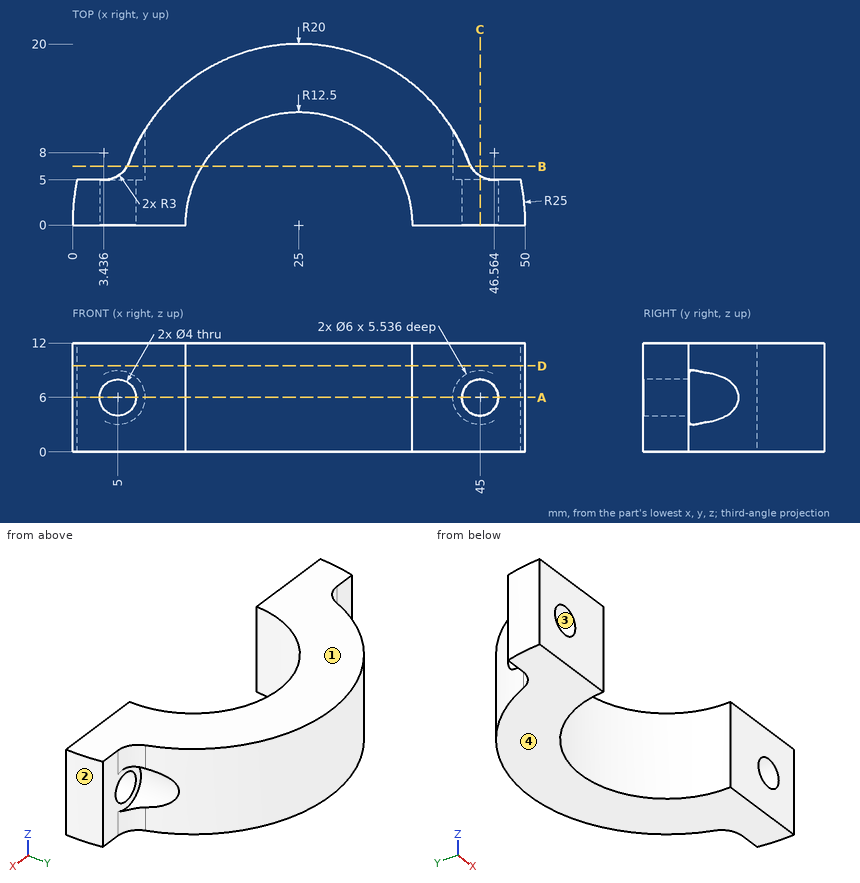
Could you check a few things on this drawing? It's one solid part, dimensions in mm from its lowest x, y, z. Coordinates: 2 decimals unless noted, no trailing zeros. Order: outer loops, then holes, each group sorted by start corner. A loop starts at its lowest first (then second) coordinate and runs counter-clockwise, first axis right, second up. Notation, with made-up numbers: (7, 40.25) -> (41, 40.25) arc R29 cw to (41, 70.25) -> close; hole circle Ø11 at (7, -39). An arc over 180 degrees is marked (long way). One line per item, written item: value. Start each with the question number.
1) If I drill on L1, parallel to X at y = 1.4, z = 6; L2, parallel to X at y = 3, z = 6 (1 decimal); L3, parallel to Z at x = 5, y = 2.1, over which ranges is the centre line in solid material (lowest first)? Write a range as [from, to].
2) Imagine slicing it at B-B on y = 6.5. List the corners of the cut face in (x, z) for me.
3) Imagine slicing it at D-D on z = 9.5. List the corners of the cut face in (x, y) for me (1 decimal).
4) I'm going to push flat-ended pins straight in: pin 1 (1 mm diameter, centred on y = 9, z = 8, fed in from +X); pin 2 (4 mm diameter, centred on x = 16.5, z = 7, fed in from -Y); pin 3 (5 mm diameter, centred on x = 11, z = 10.5, fed in from +Y). Where does each tip first touch, or does it pass through?
5) Imagine slicing it at A-A on z = 6. List the corners of the cut face in (x, y) for me (1 decimal), plus the area to 3 significant figures.
6) Imagine slicing it at C-C on x = 45. List the corners of the cut face in (y, z) for me.
7) We'd pull the mould along Z, two halves only. Please class the marked faces 1, 2, 3 and 4: +Z half, -Z half, draft (parallel to the pull), parting line (faces both ways), or undercut.
Answer list:
1. L1: x = [0.04, 3], [7, 12.58], [37.42, 43], [47, 49.96]
1. L2: x = [0.2, 3], [7, 12.9], [37.1, 43], [47, 49.8]
1. L3: z = [0, 4], [8, 12]
2. outline: (6.03, 0) -> (14.32, 0) -> (14.32, 12) -> (6.03, 12) -> (6.03, 8.82) arc R3 cw to (6.03, 3.18) -> close; (35.68, 0) -> (43.97, 0) -> (43.97, 3.18) arc R3 cw to (43.97, 8.82) -> (43.97, 12) -> (35.68, 12) -> close
3. outline: (0, 0) -> (12.5, 0) arc R12.5 cw to (37.5, 0) -> (50, 0) arc R25 ccw to (49.5, 5) -> (46.6, 5) arc R3 cw to (43.8, 7) arc R20 ccw to (6.2, 7) arc R3 cw to (3.4, 5) -> (0.5, 5) arc R25 ccw to start
4. pin 1: stops at x = 43.06
4. pin 2: stops at y = 6.78
4. pin 3: stops at y = 16.36
5. outline: (0, 0) -> (3, 0) -> (3, 5) -> (0.5, 5) arc R25 ccw to start; (7, 0) -> (12.5, 0) arc R12.5 cw to (37.5, 0) -> (43, 0) -> (43, 5) -> (42, 5) -> (42, 10.5) arc R20 ccw to (8, 10.5) -> (8, 5) -> (7, 5) -> close; (47, 0) -> (50, 0) arc R25 ccw to (49.5, 5) -> (47, 5) -> close
5. area: 378 mm2
6. outline: (0, 0) -> (5.44, 0) -> (5.44, 3) -> (5, 3) -> (5, 4) -> (0, 4) -> close; (0, 8) -> (5, 8) -> (5, 9) -> (5.44, 9) -> (5.44, 12) -> (0, 12) -> close
7. face 1: +Z half
7. face 2: draft
7. face 3: undercut
7. face 4: -Z half
